Check sheet for the modelled part. Datum: model origin and axes. Units: mm. A direction names the side the tool comes from. Give positions to 0.01 mm unless a question says otherwise; leave off trailing zeros. Write each loop counter-clockwise with the first axis right and the second up, starting at its lowest first coordinate (ties: lowest second). Pieces come first, ordered by that corner, then holes. Notation, with made-up numbers: (32, 44.5) -> (53, 44.5) arc R18 cw to (53, 52.5) -> close; hole circle Ø8 at (55, 23). An arc over 180 degrees is marked (long way). Return JSON: item names as keys, results as strings.
from build123d import *

# Parameters (mm, degrees)
SKETCH1_W           = 35
SKETCH1_H           = 45
BOSS_EXTRUDE2_DEPTH = 20
CUT_EXTRUDE1_DEPTH  = 46
CUT_EXTRUDE2_DEPTH  = 36
SKETCH5_W           = 10
SKETCH5_H           = 10
BOSS_EXTRUDE3_DEPTH = 5
CUT_EXTRUDE3_DEPTH  = 11
SKETCH7_W           = 30
SKETCH7_H           = 25
BOSS_EXTRUDE4_DEPTH = 30
SKETCH8_W           = 5
SKETCH8_H           = 10
BOSS_EXTRUDE5_DEPTH = 5
CUT_EXTRUDE4_DEPTH  = 11
SKETCH11_W          = 5
SKETCH11_H          = 45
BOSS_EXTRUDE6_DEPTH = 5
BOSS_EXTRUDE7_DEPTH = 5
CUT_EXTRUDE7_DEPTH  = 26
CUT_EXTRUDE8_DEPTH  = 26
CUT_EXTRUDE11_DEPTH = 41


with BuildPart() as part:
    # Sketch1 → Boss-Extrude2 (new body)
    with BuildSketch(Plane.XY):
        Rectangle(SKETCH1_W, SKETCH1_H)
    extrude(amount=BOSS_EXTRUDE2_DEPTH)

    # Sketch3 → Cut-Extrude1 (cut, through all)
    with BuildSketch(Plane(origin=(0, 22.5, 0), x_dir=(1, 0, 0), z_dir=(0, 1, 0))):
        Polygon((7.5, 0), (7.5, -15), (-12.5, -15), (-12.5, -5), (-7.5, -5), (-7.5, 0), align=None)
    extrude(amount=-CUT_EXTRUDE1_DEPTH, mode=Mode.SUBTRACT)

    # Sketch4 → Cut-Extrude2 (cut, through all)
    with BuildSketch(Plane(origin=(17.5, 0, 0), x_dir=(0, 0, -1), z_dir=(1, 0, 0))):
        Polygon((-5, 22.5), (-20, 7.5), (-20, 22.5), align=None)
    extrude(amount=-CUT_EXTRUDE2_DEPTH, mode=Mode.SUBTRACT)

    # Sketch5 → Boss-Extrude3 (add)
    with BuildSketch(Plane(origin=(17.5, 0, 0), x_dir=(0, 0, -1), z_dir=(1, 0, 0))):
        with Locations((-15, -17.5)):
            Rectangle(SKETCH5_W, SKETCH5_H)
    extrude(amount=BOSS_EXTRUDE3_DEPTH)

    # Sketch6 → Cut-Extrude3 (cut, through all)
    with BuildSketch(Plane(origin=(0, -12.5, 0), x_dir=(1, 0, 0), z_dir=(0, 1, 0))):
        Polygon((17.5, -20), (22.5, -15), (22.5, -20), align=None)
    extrude(amount=-CUT_EXTRUDE3_DEPTH, mode=Mode.SUBTRACT)

    # Sketch7 → Boss-Extrude4 (add)
    with BuildSketch(Plane.XY.offset(20)):
        with Locations((-2.5, -10)):
            Rectangle(SKETCH7_W, SKETCH7_H)
    extrude(amount=BOSS_EXTRUDE4_DEPTH)

    # Sketch8 → Boss-Extrude5 (add)
    with BuildSketch(Plane.XY.offset(20)):
        with Locations((15, -17.5)):
            Rectangle(SKETCH8_W, SKETCH8_H)
    extrude(amount=BOSS_EXTRUDE5_DEPTH)

    # Sketch9 → Cut-Extrude4 (cut, through all)
    with BuildSketch(Plane(origin=(0, -12.5, 0), x_dir=(1, 0, 0), z_dir=(0, 1, 0))):
        Polygon((17.5, -20), (12.5, -25), (17.5, -25), align=None)
    extrude(amount=-CUT_EXTRUDE4_DEPTH, mode=Mode.SUBTRACT)

    # Sketch11 → Boss-Extrude6 (add)
    with BuildSketch(Plane(origin=(-7.5, 0, 0), x_dir=(0, 0, -1), z_dir=(1, 0, 0))):
        with Locations((-2.5, 0)):
            Rectangle(SKETCH11_W, SKETCH11_H)
    extrude(amount=BOSS_EXTRUDE6_DEPTH)

    # Sketch12 → Boss-Extrude7 (add)
    with BuildSketch(Plane(origin=(-12.5, 0, 0), x_dir=(0, 0, -1), z_dir=(1, 0, 0))):
        Polygon((-5, 22.5), (-5, -22.5), (-15, -22.5), (-15, 12.5), align=None)
    extrude(amount=BOSS_EXTRUDE7_DEPTH)

    # Sketch13 → Cut-Extrude7 (cut, through all)
    with BuildSketch(Plane(origin=(0, 2.5, 0), x_dir=(1, 0, 0), z_dir=(0, 1, 0))):
        Polygon((12.5, -25), (-2.5, -50), (12.5, -50), align=None)
    extrude(amount=-CUT_EXTRUDE7_DEPTH, mode=Mode.SUBTRACT)

    # Sketch14 → Cut-Extrude8 (cut, through all)
    with BuildSketch(Plane(origin=(0, 2.5, 0), x_dir=(1, 0, 0), z_dir=(0, 1, 0))):
        Polygon((-17.5, -30), (-8.839745962, -35), (-17.5, -40), align=None)
    extrude(amount=-CUT_EXTRUDE8_DEPTH, mode=Mode.SUBTRACT)

    # Sketch15 → Cut-Extrude11 (cut, through all)
    with BuildSketch(Plane(origin=(-17.5, 0, 0), x_dir=(0, 0, -1), z_dir=(1, 0, 0))):
        Polygon((-20, 2.5), (-50, -17.5), (-50, 2.5), align=None)
    extrude(amount=CUT_EXTRUDE11_DEPTH, mode=Mode.SUBTRACT)


solid = part.part
(1) Set-up check for faces 5 (the flat face through (-5, 0, 5)), 6 (the flat face through (4, 3, 20)), 7 (the flat face through (7.5, 0, 7)), 8 (the flat face through (20, -12.5, 14)), 9 (the flat face through (20, -18, 10)): record each of +Z, -Z, +X, -X, +Y, -Y from which the full face is reachable in a straight line by a thin tool's end or side.
Reply:
{"face 5": "+Y, -Y", "face 6": "+Z, +X, +Y", "face 7": "-Z, +Y, -Y", "face 8": "+Z, -Z, +X, +Y", "face 9": "-Z, +X, +Y, -Y"}
(2) Release check for a two-part mould opening along X. For faces 1 (the flat face through (6.8, -13.9, 34.5)), 2 (the flat face through (12, 22.5, 2)), 3 (the flat face through (-17.5, -5, 11)), 4 (the flat face through (-7.5, 0, 10)) record: pulls with the +X half, pulls with the -X half, needs draft (parallel to the pull), parting line crosses it, or undercut.
Reply:
{"face 1": "pulls with the +X half", "face 2": "needs draft", "face 3": "pulls with the -X half", "face 4": "undercut"}
(3) Depth check by flat-ended pin: pin 1 Ø5.5 at (x, y) = (21, -16.5) entering from -Z; pin 2 Ø8 at (x, y) = (14.5, -8) entering from +Z; pin 3 Ø5.5 at (x, y) = (-4, -7.5) entering from +Z (3 decimals). Enter the tip coordinate at first touch or a pass-through.
Reply:
{"pin 1": "z = 10", "pin 2": "z = 28.33", "pin 3": "z = 39.125"}
(4) Thickness scan on L1, parallel to X at y = -9.5, z = 4.5; L2, parallel to Y at x = -12.5, z = 27.5; L3, parallel to Y at x = 10, z = 15. Record the ranges inside material, lowest first.
Reply:
{"L1": "-17.5 to -2.5, 7.5 to 17.5", "L2": "-22.5 to -2.5", "L3": "-22.5 to 12.5"}
(5) Cross-section at B-B on x = -4. Enter the section's corners in (y, z), then the cut area to 4 significant figures.
Reply:
{"outline": "(-22.5, 0) -> (22.5, 0) -> (22.5, 5) -> (-22.5, 5) -> close; (-22.5, 15) -> (12.5, 15) -> (7.5, 20) -> (2.5, 20) -> (-17.5, 50) -> (-22.5, 50) -> close", "area": "837.5 mm^2"}
(6) Cross-section at C-C on y = 3.5. Enter the section's corners in (x, z).
Reply:
{"outline": "(-17.5, 0) -> (-2.5, 0) -> (-2.5, 5) -> (-7.5, 5) -> (-7.5, 15) -> (7.5, 15) -> (7.5, 0) -> (17.5, 0) -> (17.5, 20) -> (-17.5, 20) -> close"}
(7) Cross-section at A-A on y = 16.5. Enter the section's corners in (x, z), then the cut area to 3 significant figures.
Reply:
{"outline": "(-17.5, 0) -> (-2.5, 0) -> (-2.5, 5) -> (-7.5, 5) -> (-7.5, 11) -> (-17.5, 11) -> close; (7.5, 0) -> (17.5, 0) -> (17.5, 11) -> (7.5, 11) -> close", "area": "245 mm^2"}
(8) Cross-section at D-D on x = 2. Enter the section's corners in (y, z), then the cut area to 3 significant figures.
Reply:
{"outline": "(-22.5, 15) -> (12.5, 15) -> (7.5, 20) -> (2.5, 20) -> (-12.5, 42.5) -> (-22.5, 42.5) -> close", "area": "556 mm^2"}
